For this review, take the finished solid that the model builds, in its own axes (mm). Face numbers are marked on the shaded views. A direction names the side the tool comes from. Give positions to 0.01 mm unless a question says otherwise; leave off trailing zeros. Order: outer loops, then holes, each group sorted by start corner. A loop starts at its lowest first (then second) coordinate and runs counter-clockwise, first axis right, second up. Notation, with made-up numbers: (11, 67) -> (25, 67) arc R11 ccw to (25, 85) -> close; hole circle Ø6 at (71.5, 6.25). An arc over 180 degrees is marked (long way). Return JSON: item names as keys, results as strings. Group by question number.
1) For the marked faces 1 and 2, list the 3-axis set-ups (+Z, -Z, +X, -X, +Y, -Y) from which the entire face can be reached by the end or side of a thin tool; tool diameter is ignored.
2) To check wall thickness, follow line 1 along Z through (x, y) = (4.35, 7.7); line 2 along Y through (x, z) = (3.1, -0.35); line 3 along X through (y, z) = (6.95, -0.85). State the ranges of each line that lie inside material, in increasing order.
3) Insertion check: P1, Ø1.5, axis at y = 7.5, z = -2, coming from the +X side; P2, Ø3, axis at x = 1, z = -1, coming from the +Y side. Each pin has a flat end and moves straight along its axis. Give the tip position at first contact, or say it passes through.
4) Add section A-A (z = -1.85). Give the boundary of the cut face in (x, y), then the cut area to 3 significant figures.
5) Add section B-B (z = 0.85). Give the boundary of the cut face in (x, y), then the cut area to 3 significant figures.
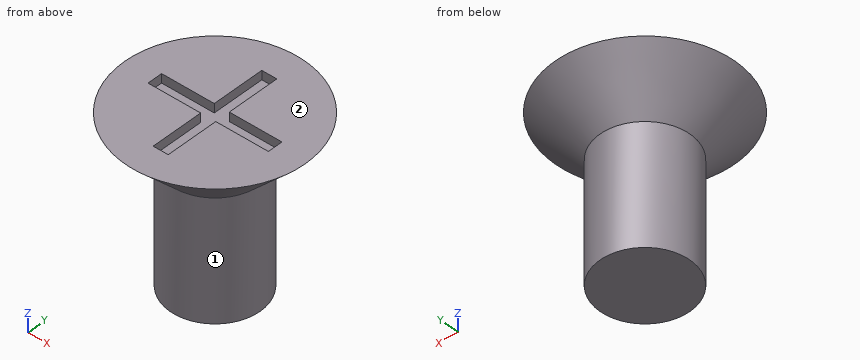
from build123d import *

# Parameters (mm, degrees)
F0_R     = 3
F1_DEPTH = 1.5
F2_SIZE  = 1.49999
F3_W     = 0.5
F3_H     = 1.75
F3_H_2   = 0.5
F3_W_2   = 1.75
F4_DEPTH = 0.3
F5_DEPTH = 4


# Not quite as in the source:
# - a fillet or chamfer is up to 0.001 mm smaller than in the source, because OpenCascade refuses the exact size


with BuildPart() as f1:
    # F0 (on Top) → F1 (new body)
    with BuildSketch(Plane.XY):
        with Locations((3.0322743114, 7.5806910172)):
            Circle(F0_R)
    extrude(amount=F1_DEPTH)

    # F2 (size 1.5 in the source; OpenCascade refuses exactly that, so slightly less here)
    f2_edges = [f1.edges().sort_by_distance(p)[0] for p in [
        (0.032274, 7.580691, 0),
    ]]
    chamfer(f2_edges, length=F2_SIZE)

    # F3 (on face) → F4 (cut)
    with BuildSketch(Plane.XY.offset(1.5)):
        with Locations((3.0322743114, 8.7056910172)):
            Rectangle(F3_W, F3_H)
        with Locations((3.0322743114, 7.5806910172)):
            Rectangle(F3_W, F3_H_2)
        with Locations((1.9072743114, 7.5806910172)):
            Rectangle(F3_W_2, F3_H_2)
        with Locations((4.1572743114, 7.5806910172)):
            Rectangle(F3_W_2, F3_H_2)
        Polygon((3.2822743114, 7.3306910172), (2.7822743114, 7.3306910172), (2.7822743114, 5.5806910172), (3.0322743114, 5.5806910172), (3.2822743114, 5.5806910172), align=None)
    extrude(amount=-F4_DEPTH, mode=Mode.SUBTRACT)

    # F5 (add): a face of the model
    f5_faces = [f1.faces().sort_by_distance(p)[0] for p in [
        (3.0322743114, 7.5806910172, 0),
    ]]
    extrude(f5_faces, amount=F5_DEPTH)


solid = f1.part
Evaluation:
{
 "1": {"face 1": "-Z", "face 2": "+Z, +X, -X, +Y, -Y"},
 "2": {"line 1": "-4 to 1.2", "line 2": "6.08 to 9.08", "line 3": "1.67 to 4.39"},
 "3": {"P1": "x = 4.53", "P2": "y = 8.98"},
 "4": {"outline": "circle Ø3 at (3.03, 7.58)", "area": "7.07 mm^2"},
 "5": {"outline": "circle Ø4.7 at (3.03, 7.58)", "area": "17.3 mm^2"}
}
